Source: CAD feature listing. Evaluate the final solid. Frame: model axes, mm. A direction names the side the tool comes from. Give positions to 0.01 mm unless a question says otherwise; leave off trailing zeros. Order: outer loops, then holes, each group sorted by start corner. A loop starts at its lowest first (then second) coordinate and runs counter-clockwise, first axis right, second up. Notation, with made-up numbers: M -29.5,27.5 L -17.5,27.5 A28 cw -17.5,54.5 Z; hole C 79.5,75.5 d5. An arc over 180 degrees is marked long. Answer as a JSON object with one key per item and string values. Group by question number.
1. Pull-direction query (Y, two-part tool) for faces 1 (the flat face through (-33.655, 1, 10)), 2 (the flat face through (32, 3.556, 10)), 3 (the flat face through (32, 5.334, 10)); classes: +Y half, -Y half, draft (parallel to the pull), parting line (faces both ways), or undercut.
2. Section query C-C (y = 1). Output: boundary loops of the cut face in (x, z) (3 decimals), plus the area to 3 significant figures.
3. Section query A-A (z = 15.5). Output: boundary loops of the cut face in (x, y) (3 decimals).
4. Pin query (flat end, axial travel): P1, Ø1.6, axis at x = -4.5, y = 0.5, coming from the +Z side; P2, Ø1, axis at x = -24, z = 4.5, coming from the +Y side. Return the tip coordinate at first contact, or that it passes through.
5. Material intervals for L1, parallel to X at y = 1.1, z = 15.75 (3 decimals); L2, parallel to X at y = 4.9, z = 4 (3 decimals); L3, parallel to X at y = 2.75, z = 7.25 (3 decimals), sorted ascending. Write a range as [from, to].
6. Section query B-B (x = 4). Output: boundary loops of the cut face in (y, z), plus the area to 3 significant figures.
7. Set-up query: faces 4 (the flat face through (-0.2, 2.032, 4.7)), 5 (the flat face through (0, 4, 5.08)), 6 (the flat face through (-32, 1.778, 10)), 7 (the flat face through (31.115, 3, 10)). Return all of +Z, -Z, +X, -X, +Y, -Y with unobstructed straight access to the full face (end or side cutting, diameter ignored); none if empty.
from build123d import *

# Parameters (mm, degrees)
F1_DEPTH = 20.32
F2_W     = 30.988
F2_H     = 5.334
F3_DEPTH = 12.7
F4_W     = 30.988
F4_H     = 1.27
F5_DEPTH = 3.556
F7_DEPTH = 5.334


with BuildPart() as f1:
    # F0 (on Top) → F1 (new body)
    with BuildSketch(Plane.XY):
        Polygon((-31.115, 1.778), (-33.655, 1.778), (-33.655, 0), (33.655, 0), (33.655, 1.778), (31.115, 1.778), (31.115, 3.556), (33.655, 3.556), (33.655, 5.334), (29.845, 5.334), (28.575, 3.556), (16.51, 3.556), (16.51, 5.334), (-16.51, 5.334), (-16.51, 3.556), (-28.575, 3.556), (-29.845, 5.334), (-33.655, 5.334), (-33.655, 3.556), (-31.115, 3.556), align=None)
    extrude(amount=F1_DEPTH)

    # F2 (on face) → F3 (cut)
    with BuildSketch(Plane.XY.offset(20.32)):
        with Locations((0, 2.667)):
            Rectangle(F2_W, F2_H)
    extrude(amount=-F3_DEPTH, mode=Mode.SUBTRACT)

    # F4 (on face) → F5 (cut)
    with BuildSketch(Plane.XY.offset(7.62)):
        with Locations((0, 2.667)):
            Rectangle(F4_W, F4_H)
    extrude(amount=-F5_DEPTH, mode=Mode.SUBTRACT)

    # F6 (on face) → F7 (cut, through all)
    with BuildSketch(Plane.XZ):
        Polygon((15.494, 7.62), (-15.494, 7.62), (-9.144, 5.08), (9.144, 5.08), align=None)
    extrude(amount=-F7_DEPTH, mode=Mode.SUBTRACT)


solid = f1.part
Answer sheet:
{
 "1": {"face 1": "draft", "face 2": "undercut", "face 3": "+Y half"},
 "2": {"outline": "M -33.655,0 L 33.655,0 L 33.655,20.32 L 15.494,20.32 L 15.494,7.62 L 9.144,5.08 L -9.144,5.08 L -15.494,7.62 L -15.494,20.32 L -33.655,20.32 Z", "area": "912 mm^2"},
 "3": {"outline": "M -33.655,0 L -15.494,0 L -15.494,5.334 L -16.51,5.334 L -16.51,3.556 L -28.575,3.556 L -29.845,5.334 L -33.655,5.334 L -33.655,3.556 L -31.115,3.556 L -31.115,1.778 L -33.655,1.778 Z; M 15.494,0 L 33.655,0 L 33.655,1.778 L 31.115,1.778 L 31.115,3.556 L 33.655,3.556 L 33.655,5.334 L 29.845,5.334 L 28.575,3.556 L 16.51,3.556 L 16.51,5.334 L 15.494,5.334 Z"},
 "4": {"P1": "z = 5.08", "P2": "y = 3.56"},
 "5": {"L1": "[-33.655, -15.494], [15.494, 33.655]", "L2": "[-33.655, -29.535], [-16.51, 16.51], [29.535, 33.655]", "L3": "[-31.115, -15.494], [15.494, 31.115]"},
 "6": {"outline": "M 0,0 L 5.33,0 L 5.33,5.08 L 3.3,5.08 L 3.3,4.06 L 2.03,4.06 L 2.03,5.08 L 0,5.08 Z", "area": "25.8 mm^2"},
 "7": {"face 4": "+Z", "face 5": "+Z, +Y, -Y", "face 6": "+Z, -Z, -X", "face 7": "+Z, -Z, +X"}
}
